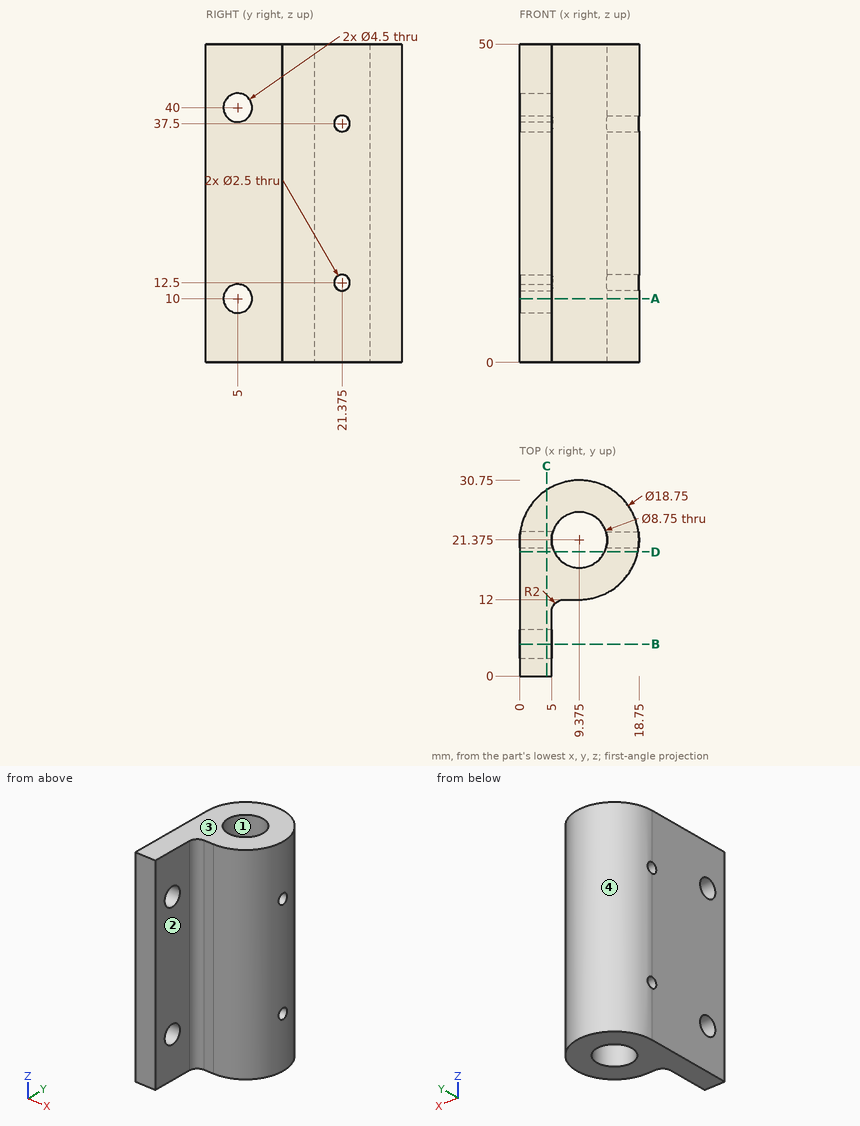
Input: dimensioned drawing with shaded views. Units: mm. Origin: part minimum x, y, z. Coordinates: 2 decimals unless noted, no trailing zeros. Loops run counter-clockwise (first coordinate to the right, second up) from the corner with the lowest first, then second, coordinate; pieces in that order, holes last. Notation, with made-up numbers: M -14,59.25 L 1,59.25 A20 cw 1,89.25 Z; hole C 73,46 d3. An arc over 180 degrees is marked long. Put each result on its own line as item: value.
(1) Cut plane C-C on x = 4.25. Return the cut outline in (y, z) (3 decimals).
Answer sheet:
outline: M 0,0 L 29.225,0 L 29.225,50 L 0,50 Z; hole C 5,10 d4.5; hole C 5,40 d4.5; hole C 21.375,12.5 d2.5; hole C 21.375,37.5 d2.5
(2) Material intervals for probe 1 along Z at (x, y) = (3, 5); probe 2 along Y at (x, z) = (11, 14.5); probe 3 along Y at (x, z) = (13, 15.5), sorted ascending.
Answer sheet:
probe 1: z = 0 to 7.75, 12.25 to 37.75, 42.25 to 50
probe 2: y = 12.14 to 17.31, 25.44 to 30.61
probe 3: y = 12.73 to 18.93, 23.82 to 30.02
(3) Cut plane D-D on y = 19.5. Return the cut outline in (x, z), then the cut area to 3 significant figures.
Answer sheet:
outline: M 0,0 L 5.42,0 L 5.42,50 L 0,50 Z; M 13.33,0 L 18.56,0 L 18.56,50 L 13.33,50 Z
area: 533 mm^2
(4) Cut plane A-A on z = 10. Return the cut outline in (x, y) (3 decimals), then the cut area to 3 significant figures.
Answer sheet:
outline: M 0,0 L 5,0 L 5,2.75 L 0,2.75 Z; M 0,7.25 L 5,7.25 L 5,10 A2 cw 7,12 L 9.375,12 A9.375 ccw long 0,21.375 Z; hole C 9.375,21.375 d8.75
area: 273 mm^2
(5) First-contact query: pin 1 (10 mm diameter, centred on y = 21, z = 41.5, fed in from +X); pin 2 (4 mm diameter, centred on x = 15, z = 16.5, fed in from +Y); pin 3 (4 mm diameter, centred on y = 5, z = 43.5, fed in from +X); pin 4 (0.7 mm diameter, centred on x = 8, z = 32.5, fed in from -Y). Flat tips, straight axial feed; report the tip coordinate or a pass-through.
Answer sheet:
pin 1: stops at x = 18.75
pin 2: stops at y = 30.02
pin 3: stops at x = 5
pin 4: stops at y = 12
(6) Cut plane B-B on y = 5. Return the cut outline in (x, z), then the cut area to 3 significant figures.
Answer sheet:
outline: M 0,0 L 5,0 L 5,7.75 L 0,7.75 Z; M 0,12.25 L 5,12.25 L 5,37.75 L 0,37.75 Z; M 0,42.25 L 5,42.25 L 5,50 L 0,50 Z
area: 205 mm^2
(7) Draft query along X for the marked faces 1, 2, 3 and 4. Return one class per face: pulls with the +X half, pulls with the -X half, needs draft (parallel to the pull), parting line crosses it, or undercut.
Answer sheet:
face 1: undercut
face 2: pulls with the +X half
face 3: needs draft
face 4: parting line crosses it
